```python
from build123d import *

# Parameters (mm, degrees)
F0_R            = 42.0966561171
F1_DEPTH        = 25.4
F3_DEPTH        = 25.401
F3_COPIES_COUNT = 3
F4_R            = 2.54
F5_R            = 2.54


# Not quite as in the source:
# - a pattern or mirror of a feature is missing from the dataset's text; its kind, count and spacing are read off the source's solid


with BuildPart() as f1:
    # F0 (on Front) → F1 (new body)
    with BuildSketch(Plane.XZ):
        Circle(F0_R)
    extrude(amount=F1_DEPTH)

    # F2 (on face) → F3 (cut, through all)
    with BuildSketch(Plane.XZ.offset(25.4)):
        Polygon((-18.881084953, 4.9543602206), (-8.2484530285, 8.3401026204), (-5.8642759952, 19.241103176), (-14.1127308863, 26.7563613318), (-24.7453628108, 23.3706189319), (-27.1295398441, 12.4696183764), align=None)
    f3 = extrude(amount=-F3_DEPTH, mode=Mode.SUBTRACT)

    # F3_copies: F3 ×3 about axis
    f3_copies_axis = Axis((0, 0, 0), (0, 1, 0))
    for i in range(1, F3_COPIES_COUNT):
        add(f3.rotate(f3_copies_axis, i * 360 / F3_COPIES_COUNT), mode=Mode.SUBTRACT)

    # F4
    f4_edges = [f1.edges().sort_by_distance(p)[0] for p in [
        (-42.096656, -25.4, 0),
    ]]
    fillet(f4_edges, radius=F4_R)

    # F5
    f5_edges = [f1.edges().sort_by_distance(p)[0] for p in [
        (-42.096656, 0, 0),
    ]]
    fillet(f5_edges, radius=F5_R)


solid = f1.part
```
Work out the finished part from the listing and answer in its coordinate system (mm). A direction names the side the tool comes from. Round coordinates to 2 decimals unless told otherwise and drop trailing zeros. Write each loop counter-clockwise with the first axis right and the second up, starting at its lowest first coordinate (ties: lowest second). Pieces come first, ordered by that corner, then holes.
1) Consider probe 1 along X at (y, z) = (-10, -24); probe 2 along Z at (x, y) = (-17, -3.25); probe 3 along Z at (x, y) = (16.5, -15). Determine where each line is inside the solid, lowest interval first.
2) A cutting plane is placed at C-C on x = 0. Determine the outline of the cut face in (y, z).
3) Which of the six approach directions +Z, -Z, +X, -X, +Y, -Y give full straight-line access (tool end or side, diameter ignored) to faces 1 (the face through (-13.639, -12.878, 6.624)), 2 (the face through (-1, 0, 1))?
4) A cutting plane is placed at B-B on y = -11.5. Determine the outline of the cut face in (x, z), and give its area (3 significant figures).
5) A cutting plane is placed at A-A on z = 0. Determine the outline of the cut face in (x, y), and give its area (3 significant figures).
6) Flat-ended cylindrical pins translate along their axes: P1, Ø5, axis at x = -18.5, y = -20.5, coming from the -Z side; P2, Ø2, axis at x = 20, y = -22, coming from the -Z side (3 decimals); P3, Ø8, axis at y = -14.5, z = 21, coming from the -X side. Find the tip coordinate at first contact, or state that the pin passes through.
Entries:
1. probe 1: x = -34.59 to -15.77, 4.02 to 34.59
1. probe 2: z = -38.51 to 5.55, 25.84 to 38.51
1. probe 3: z = -38.73 to -1.72, 14.76 to 38.73
2. outline: (-25.4, -39.56) arc R2.54 ccw to (-22.86, -42.1) - (-2.54, -42.1) arc R2.54 ccw to (0, -39.56) - (0, -30.61) - (-25.4, -30.61) - close; (-25.4, -14.14) - (0, -14.14) - (0, 39.56) arc R2.54 ccw to (-2.54, 42.1) - (-22.86, 42.1) arc R2.54 ccw to (-25.4, 39.56) - close
3. face 1: +Y, -Y
3. face 2: +Z, -Z, +X, -X, +Y
4. outline: circle Ø84.19 at (0, 0); hole (-27.13, 12.47) - (-18.88, 4.95) - (-8.25, 8.34) - (-5.86, 19.24) - (-14.11, 26.76) - (-24.75, 23.37) - close; hole (-16.12, -25.6) - (-7.87, -33.12) - (2.77, -29.73) - (5.15, -18.83) - (-3.1, -11.31) - (-13.73, -14.7) - close; hole (11.35, 2.97) - (19.6, -4.54) - (30.23, -1.16) - (32.61, 9.74) - (24.36, 17.26) - (13.73, 13.87) - close
4. area: 4,600 mm2
5. outline: (-42.1, -22.86) arc R2.54 ccw to (-39.56, -25.4) - (14.61, -25.4) - (14.61, 0) - (-39.56, 0) arc R2.54 ccw to (-42.1, -2.54) - close; (30.48, -25.4) - (39.56, -25.4) arc R2.54 ccw to (42.1, -22.86) - (42.1, -2.54) arc R2.54 ccw to (39.56, 0) - (30.48, 0) - close
5. area: 1,730 mm2
6. P1: stops at z = -38.94
6. P2: stops at z = -37.565
6. P3: stops at x = -38.51
